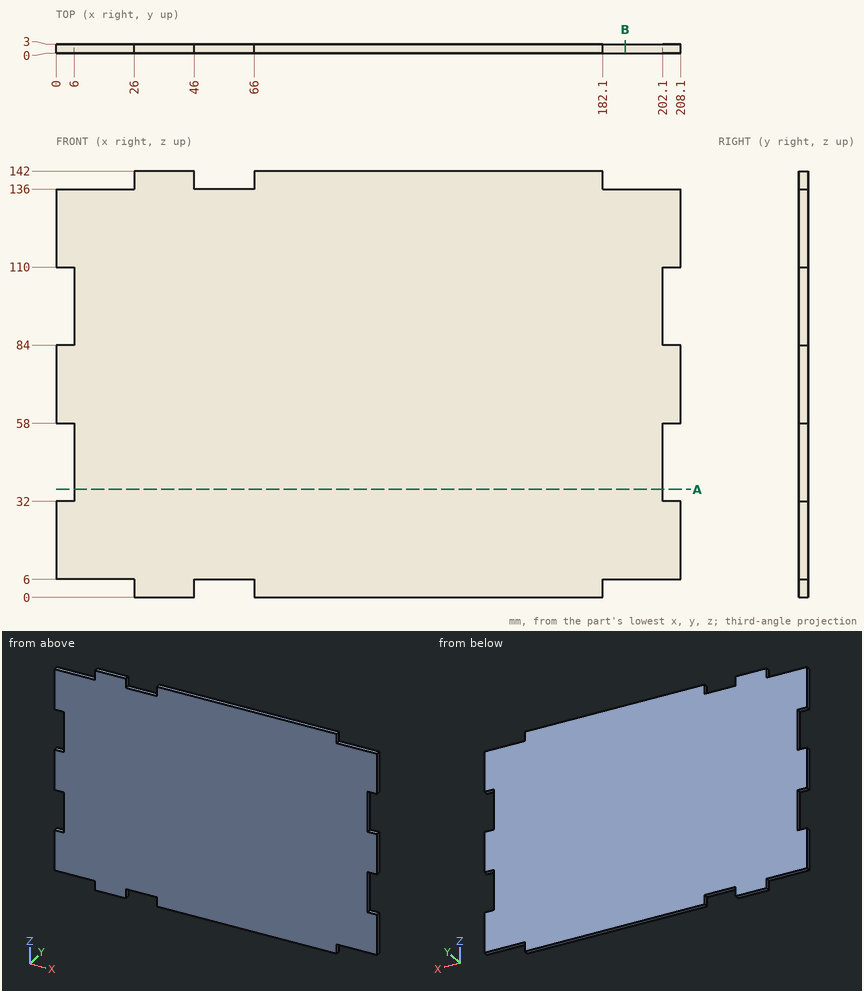
Design review of the part shown in the three views and the two pictorial views. Dimensions are in mm from the part's minimum x, y and z. Round coordinates to 2 decimals unless told otherwise and drop trailing zeros. Write each loop counter-clockwise with the first axis right and the second up, starting at its lowest first coordinate (ties: lowest second). Pieces come first, ordered by that corner, then holes.
1) Take a section at A-A on z = 36. Give the boundary of the cut face in (x, y).
Answer below:
outline: (6, 0) - (202.1, 0) - (202.1, 3) - (6, 3) - close
2) For line 1 along Z through (x, y) = (62.5, 0.25); line 2 along X through (y, z) = (2.3, 56.5), list the stretches that pass through material, from the lowest coordinate up.
Answer below:
line 1: z = 6 to 136
line 2: x = 6 to 202.1
3) Insertion check: pin 1 Ø1.5 at (x, y) = (57.5, 1) entering from +Z; pin 2 Ø0.9 at (y, z) = (1.5, 3.5) entering from -X; pin 3 Ø0.9 at (x, y) = (206.5, 1.5) entering from -Z. Each pin has a flat end and moves straight along its axis. Give the tip position at first contact, or say it passes through.
Answer below:
pin 1: stops at z = 136
pin 2: stops at x = 26
pin 3: stops at z = 6
4) Take a section at B-B on x = 189.5. Give the boundary of the cut face in (y, z), then the cut area to 3 significant figures.
Answer below:
outline: (0, 6) - (3, 6) - (3, 136) - (0, 136) - close
area: 390 mm2
